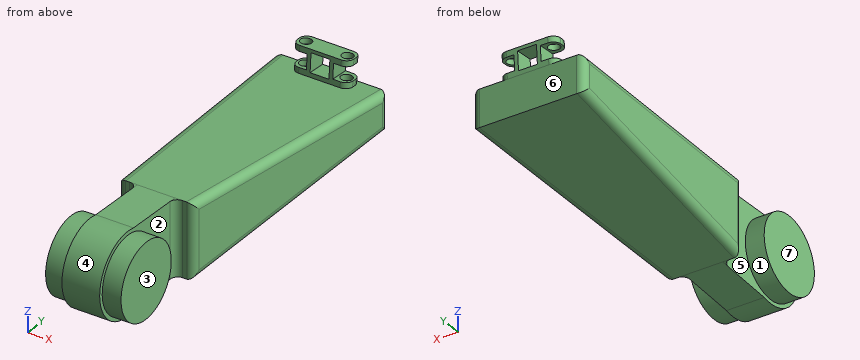
```python
from build123d import *

# Parameters (mm, degrees)
SALIENTE_EXTRUIR1_DEPTH = 5
CROQUIS5_R              = 10
SALIENTE_EXTRUIR2_DEPTH = 10
CROQUIS6_R              = 1.5
SALIENTE_EXTRUIR3_DEPTH = 7
CROQUIS7_W              = 4
CROQUIS7_H              = 4
CORTAR_EXTRUIR1_DEPTH   = 5
REDONDEO1_R             = 2
CROQUIS8_W              = 5
CROQUIS8_H              = 5
CORTAR_EXTRUIR2_DEPTH   = 10


with BuildPart() as part:
    # Croquis2 → Recubrir1 section 0
    with BuildSketch(Plane(origin=(0, 70, 0), x_dir=(1, 0, 0), z_dir=(0, 1, 0))):
        with BuildLine():
            Line((15, -5), (-15, -5))
            Line((-15, -5), (-15, 5))
            Line((-15, 5), (15, 5))
            Line((15, 5), (15, -5))
        make_face()
    # Croquis1 → Recubrir1 section 1
    with BuildSketch(Plane(origin=(0, 0, 0), x_dir=(1, 0, 0), z_dir=(0, 1, 0))):
        with BuildLine():
            Line((10, -10), (-10, -10))
            Line((-10, -10), (-10, 10))
            Line((-10, 10), (10, 10))
            Line((10, 10), (10, -10))
        make_face()
    loft()

    # Croquis4 → Saliente-Extruir1 (add, symmetric)
    with BuildSketch(Plane(origin=(0, 0, 0), x_dir=(0, 0, -1), z_dir=(1, 0, 0))):
        with BuildLine():
            Line((-10, 0), (-10.71921501, -16.530500138))
            ThreePointArc((-10.71921501, -16.530500138), (0, -30), (10.71921501, -16.530500138))
            Line((10.71921501, -16.530500138), (10, 0))
            Line((10, 0), (-10, 0))
        make_face()
    extrude(amount=SALIENTE_EXTRUIR1_DEPTH, both=True)

    # Croquis5 → Saliente-Extruir2 (add, symmetric)
    with BuildSketch(Plane(origin=(0, 0, 0), x_dir=(0, 0, -1), z_dir=(1, 0, 0))):
        with Locations((0, -19)):
            Circle(CROQUIS5_R)
    extrude(amount=SALIENTE_EXTRUIR2_DEPTH, both=True)

    # Croquis6 → Saliente-Extruir3 (add)
    with BuildSketch(Plane(origin=(0, 0.710659898, 9.949238579), x_dir=(1, 0, 0), z_dir=(0, 0.07124704998790965, 0.997458699830735))):
        with BuildLine():
            Line((-5.5, 64.465873738), (5.5, 64.465873738))
            ThreePointArc((5.5, 64.465873738), (6.914213562, 65.051660176), (7.5, 66.465873738))
            Line((7.5, 66.465873738), (7.5, 67.465873738))
            ThreePointArc((7.5, 67.465873738), (6.914213562, 68.880087301), (5.5, 69.465873738))
            Line((5.5, 69.465873738), (-5.5, 69.465873738))
            ThreePointArc((-5.5, 69.465873738), (-6.914213562, 68.880087301), (-7.5, 67.465873738))
            Line((-7.5, 67.465873738), (-7.5, 66.465873738))
            ThreePointArc((-7.5, 66.465873738), (-6.914213562, 65.051660176), (-5.5, 64.465873738))
        make_face()
        with Locations(Location((-5.5, 66.965873738, 0), (0, 0, 90))):
            Circle(CROQUIS6_R, mode=Mode.SUBTRACT)
        with Locations(Location((5.5, 66.965873738, 0), (0, 0, 90))):
            Circle(CROQUIS6_R, mode=Mode.SUBTRACT)
    extrude(amount=SALIENTE_EXTRUIR3_DEPTH)

    # Croquis7 → Cortar-Extruir1 (cut, symmetric)
    with BuildSketch(Plane(origin=(0, 69.289340102, -4.949238579), x_dir=(1, 0, 0), z_dir=(0, 0.997458699830735, -0.07124704998790966))):
        with Locations((-5.5, -13.474586998)):
            Rectangle(CROQUIS7_W, CROQUIS7_H)
        with Locations((5.5, -13.474586998)):
            Rectangle(CROQUIS7_W, CROQUIS7_H)
    extrude(amount=CORTAR_EXTRUIR1_DEPTH, both=True, mode=Mode.SUBTRACT)

    # Redondeo1
    # the kernel refuses this fillet: 2 mm, written as the material it adds along each edge
    with BuildSketch(Plane(origin=(-5, 0, -15), x_dir=(-1, 0, 0), z_dir=(0, 0, 1))) as redondeo1_piece_1_section:
        with BuildLine():
            CenterArc((REDONDEO1_R, REDONDEO1_R), REDONDEO1_R, 180, 90)
            Line((0, REDONDEO1_R), (0, 0))
            Line((0, 0), (REDONDEO1_R, 0))
        make_face()
    redondeo1_piece_1 = extrude(amount=30, mode=Mode.PRIVATE)
    redondeo1_piece_1 = split(redondeo1_piece_1, bisect_by=Plane(origin=(-5.45231098, -0.018481015, 10.000804079), z_dir=(0, -0.043467241760335076, -0.999054852795255)), keep=Keep.TOP, mode=Mode.PRIVATE)
    redondeo1_piece_1 = split(redondeo1_piece_1, bisect_by=Plane(origin=(-5.45231098, -0.018481001, -10.000804078), z_dir=(0, -0.04346724176032877, 0.9990548527952553)), keep=Keep.TOP, mode=Mode.PRIVATE)
    add(redondeo1_piece_1)
    with BuildSketch(Plane(origin=(5, 0, -15), x_dir=(1, 0, 0), z_dir=(0, 0, 1))) as redondeo1_piece_2_section:
        with BuildLine():
            CenterArc((REDONDEO1_R, -REDONDEO1_R), REDONDEO1_R, 90, 90)
            Line((0, -REDONDEO1_R), (0, 0))
            Line((0, 0), (REDONDEO1_R, 0))
        make_face()
    redondeo1_piece_2 = extrude(amount=30, mode=Mode.PRIVATE)
    redondeo1_piece_2 = split(redondeo1_piece_2, bisect_by=Plane(origin=(5.45231098, -0.018481001, 10.000804078), z_dir=(0, -0.043467241760335076, -0.999054852795255)), keep=Keep.TOP, mode=Mode.PRIVATE)
    redondeo1_piece_2 = split(redondeo1_piece_2, bisect_by=Plane(origin=(5.45231098, -0.018481015, -10.000804079), z_dir=(0, -0.04346724176032877, 0.9990548527952553)), keep=Keep.TOP, mode=Mode.PRIVATE)
    add(redondeo1_piece_2)
    # the kernel refuses this fillet: 2 mm, written as the material it takes off along each edge
    with BuildSketch(Plane(origin=(15, 70, -10.369881731), x_dir=(-1, 0, 0), z_dir=(0, 0, 1))) as redondeo1_2_piece_1:
        with BuildLine():
            CenterArc((REDONDEO1_R * 1.07397634626, REDONDEO1_R), REDONDEO1_R, 175.91438322, 94.08561678)
            Line((REDONDEO1_R * 0.0765176464277, REDONDEO1_R * 1.07124704999), (0, 0))
            Line((0, 0), (REDONDEO1_R * 1.07397634626, 0))
        make_face()
    extrude(amount=20.739763463, mode=Mode.SUBTRACT)
    with BuildSketch(Plane(origin=(15.357142857, 75, -4.642857143), x_dir=(-0.9974715509474419, 0.07088630311301622, 0.00506330736521557), z_dir=(-0.07106690545187021, -0.9949366763261821, -0.07106690545187017)), Plane(origin=(-15.357142857, 75, 4.642857143), x_dir=(0.9974715509474419, 0.07088630311301611, -0.005063307365215563), z_dir=(0.0710669054518701, -0.9949366763261821, 0.07106690545187014))) as redondeo1_2_piece_2:
        with BuildLine():
            CenterArc((REDONDEO1_R * 1.00508909139, -REDONDEO1_R), REDONDEO1_R, 90, 90.290842769)
            Line((REDONDEO1_R * 0.0051019750832, -REDONDEO1_R * 1.00507614213), (0, 0))
            Line((0, 0), (REDONDEO1_R * 1.00508909139, 0))
        make_face()
    extrude(amount=80.407127311, mode=Mode.SUBTRACT)
    with BuildSketch(Plane(origin=(10, 0, -14.655596017), x_dir=(-1, 0, 0), z_dir=(0, 0, 1)), Plane(origin=(-10, 0, 14.655596017), x_dir=(1, 0, 0), z_dir=(0, 0, -1))) as redondeo1_2_piece_3:
        with BuildLine():
            CenterArc((REDONDEO1_R * 0.931119203401, -REDONDEO1_R), REDONDEO1_R, 90, 85.91438322)
            Line((-REDONDEO1_R * 0.0663394964294, -REDONDEO1_R * 0.928752950012), (0, 0))
            Line((0, 0), (REDONDEO1_R * 0.931119203401, 0))
        make_face()
    extrude(amount=29.311192034, mode=Mode.SUBTRACT)
    with BuildSketch(Plane(origin=(15.357142857, 75, 4.642857143), x_dir=(-0.9974715509474419, 0.07088630311301623, -0.005063307365215571), z_dir=(-0.07106690545187021, -0.9949366763261821, 0.07106690545187014)), Plane(origin=(-15.357142857, 75, -4.642857143), x_dir=(0.9974715509474419, 0.07088630311301615, 0.005063307365215123), z_dir=(0.0710669054518701, -0.9949366763261821, -0.07106690545187017))) as redondeo1_2_piece_4:
        with BuildLine():
            CenterArc((REDONDEO1_R * 1.00508909139, REDONDEO1_R), REDONDEO1_R, 179.709157231, 90.290842769)
            Line((REDONDEO1_R * 0.0051019750832, REDONDEO1_R * 1.00507614213), (0, 0))
            Line((0, 0), (REDONDEO1_R * 1.00508909139, 0))
        make_face()
    extrude(amount=80.407127311, mode=Mode.SUBTRACT)
    with BuildSketch(Plane(origin=(-15, 70, 10.369881731), x_dir=(0.07124704998790952, -0.997458699830735, 0), z_dir=(0, 0, -1))) as redondeo1_2_piece_5:
        with BuildLine():
            CenterArc((REDONDEO1_R * 1.07397634626, -REDONDEO1_R), REDONDEO1_R, 90, 94.08561678)
            Line((REDONDEO1_R * 0.0765176464277, -REDONDEO1_R * 1.07124704999), (0, 0))
            Line((0, 0), (REDONDEO1_R * 1.07397634626, 0))
        make_face()
    extrude(amount=20.739763463, mode=Mode.SUBTRACT)

    # Croquis8 → Cortar-Extruir2 (cut)
    with BuildSketch(Plane(origin=(0, 69.289340102, -4.949238579), x_dir=(1, 0, 0), z_dir=(0, 0.997458699830735, -0.07124704998790966))):
        with Locations((0, -13.621474852)):
            Rectangle(CROQUIS8_W, CROQUIS8_H)
    extrude(amount=-CORTAR_EXTRUIR2_DEPTH, mode=Mode.SUBTRACT)


solid = part.part
```
Design review of the part built by this model. Coordinates are the model's own, in mm. Face numbers are marked on the shaded views. A direction names the side the tool comes from. Coordinates: 2 decimals unless noted, no trailing zeros. Order: outer loops, then holes, each group sorted by start corner. A loop starts at its lowest first (then second) coordinate and runs counter-clockwise, first axis right, second up. Notation, with made-up numbers: (-27, 30) - (21, 30) arc R27 ccw to (21, 47) - close; hole circle Ø9 at (-6.75, 81). An arc over 180 degrees is marked (long way). One line per question, with ' | ' between items.
Q1. For the marked faces 1, 2, 3 and 4, list the 3-axis set-ups (+Z, -Z, +X, -X, +Y, -Y) from which the entire face can be reached by the end or side of a thin tool; tool diameter is ignored.
Answer key:
face 1: -X | face 2: +X | face 3: +Z, -Z, +X, -Y | face 4: +X, -X
Q2. The part is to be moulded in two halves that separate along Y. For the marked faces 5, 6 and 7, say which applies: +Y half, -Y half, draft (parallel to the pull), parting line (faces both ways), or undercut.
Answer key:
face 5: undercut | face 6: +Y half | face 7: draft
Q3. Clearance check with flat-ended pins moving along their axes: pin 1 Ø10 at (y, z) = (-23, -4) entering from +X; pin 2 Ø11 at (y, z) = (-11.5, 1.5) entering from -X; pin 3 Ø4 at (y, z) = (57.5, -7) entering from -X. State where each tip first meets the part, or that it passes through.
Answer key:
pin 1: stops at x = 10 | pin 2: stops at x = -10 | pin 3: stops at x = -13.77
Q4. Consider section A-A, the plane y = -19. Give the boundary of the cut face in (x, z), then the cut area to 3 significant figures.
Answer key:
outline: (-10, -10) - (-5, -10) - (-5, -11) - (5, -11) - (5, -10) - (10, -10) - (10, 10) - (5, 10) - (5, 11) - (-5, 11) - (-5, 10) - (-10, 10) - close | area: 420 mm2
Q5. To check wall thickness, follow line 1 along X through (y, z) = (40, 4.75); line 2 along Z through (x, y) = (6.5, 30); line 3 along X through (y, z) = (-7, -0.25). State the ranges of each line that lie inside material, in increasing order.
Answer key:
line 1: x = -12.86 to 12.86 | line 2: z = -7.86 to 7.86 | line 3: x = -5 to 5
